```python
from build123d import *

# Parameters (mm, degrees)
F0_W     = 1400
F0_H     = 700
F0_W_2   = 420.8995199203
F0_H_2   = 620
F0_W_3   = 420
F0_H_3   = 350
F0_W_4   = 400
F0_H_4   = 600
F0_H_5   = 50
F1_DEPTH = 25
F2_DEPTH = 500
F3_START = 490
F3_DEPTH = 10


with BuildPart() as f1:
    # F0 (on Front) → F1 (new body)
    with BuildSketch(Plane.XZ):
        with Locations((0, 350)):
            Rectangle(F0_W, F0_H)
        with Locations((-450.4497599602, 350)):
            Rectangle(F0_W_2, F0_H_2, mode=Mode.SUBTRACT)
        with Locations((0, 350)):
            Rectangle(F0_W_3, F0_H_2, mode=Mode.SUBTRACT)
        with Locations((450, 350)):
            Rectangle(F0_W_3, F0_H_2, mode=Mode.SUBTRACT)
        with Locations((0, 875)):
            Rectangle(F0_W, F0_H_3)
        with Locations((0, 1275)):
            Rectangle(F0_W, F0_H_3)
        with Locations((0, 1675)):
            Rectangle(F0_W, F0_H_3)
        with Locations((-450.4497599602, 350)):
            Rectangle(F0_W_2, F0_H_2)
        with Locations((-450, 350)):
            Rectangle(F0_W_4, F0_H_4, mode=Mode.SUBTRACT)
        with Locations((450, 350)):
            Rectangle(F0_W_3, F0_H_2)
        with Locations((450, 350)):
            Rectangle(F0_W_4, F0_H_4, mode=Mode.SUBTRACT)
        with Locations((0, 350)):
            Rectangle(F0_W_3, F0_H_2)
        with Locations((0, 350)):
            Rectangle(F0_W_4, F0_H_4, mode=Mode.SUBTRACT)
        with Locations((450, 350)):
            Rectangle(F0_W_4, F0_H_4)
        with Locations((0, 350)):
            Rectangle(F0_W_4, F0_H_4)
        with Locations((-450, 350)):
            Rectangle(F0_W_4, F0_H_4)
        with Locations((0, 1075)):
            Rectangle(F0_W, F0_H_5)
        with Locations((0, 1475)):
            Rectangle(F0_W, F0_H_5)
        with Locations((0, 1875)):
            Rectangle(F0_W, F0_H_5)
    extrude(amount=F1_DEPTH)

    # F0 (on Front) → F2 (join)
    with BuildSketch(Plane.XZ):
        with Locations((0, 350)):
            Rectangle(F0_W, F0_H)
        with Locations((-450.4497599602, 350)):
            Rectangle(F0_W_2, F0_H_2, mode=Mode.SUBTRACT)
        with Locations((0, 350)):
            Rectangle(F0_W_3, F0_H_2, mode=Mode.SUBTRACT)
        with Locations((450, 350)):
            Rectangle(F0_W_3, F0_H_2, mode=Mode.SUBTRACT)
        with Locations((-450.4497599602, 350)):
            Rectangle(F0_W_2, F0_H_2)
        with Locations((-450, 350)):
            Rectangle(F0_W_4, F0_H_4, mode=Mode.SUBTRACT)
        with Locations((450, 350)):
            Rectangle(F0_W_3, F0_H_2)
        with Locations((450, 350)):
            Rectangle(F0_W_4, F0_H_4, mode=Mode.SUBTRACT)
        with Locations((0, 350)):
            Rectangle(F0_W_3, F0_H_2)
        with Locations((0, 350)):
            Rectangle(F0_W_4, F0_H_4, mode=Mode.SUBTRACT)
        with Locations((-450, 350)):
            Rectangle(F0_W_4, F0_H_4)
        with Locations((0, 350)):
            Rectangle(F0_W_4, F0_H_4)
        with Locations((450, 350)):
            Rectangle(F0_W_4, F0_H_4)
        with Locations((0, 1875)):
            Rectangle(F0_W, F0_H_5)
        with Locations((0, 1475)):
            Rectangle(F0_W, F0_H_5)
        with Locations((0, 1075)):
            Rectangle(F0_W, F0_H_5)
    extrude(amount=F2_DEPTH)

    # F0 (on Front) → F3 (cut)
    with BuildSketch(Plane.XZ.offset(F3_START)):
        with Locations((450, 350)):
            Rectangle(F0_W_3, F0_H_2)
        with Locations((450, 350)):
            Rectangle(F0_W_4, F0_H_4, mode=Mode.SUBTRACT)
        with Locations((0, 350)):
            Rectangle(F0_W_3, F0_H_2)
        with Locations((0, 350)):
            Rectangle(F0_W_4, F0_H_4, mode=Mode.SUBTRACT)
        with Locations((-450.4497599602, 350)):
            Rectangle(F0_W_2, F0_H_2)
        with Locations((-450, 350)):
            Rectangle(F0_W_4, F0_H_4, mode=Mode.SUBTRACT)
    extrude(amount=F3_DEPTH, mode=Mode.SUBTRACT)


solid = f1.part
```
The listing builds one solid part. Answer for the finished solid, in the listing's coordinates (mm). A direction names the side the tool comes from. Round coordinates to 2 decimals unless told otherwise and drop trailing zeros. Loops run counter-clockwise (first coordinate to the right, second up) from the corner with the lowest first, then second, coordinate; pieces in that order, holes last.
Q1. Which of the six approach directions +Z, -Z, +X, -X, +Y, -Y give full straight-line access (tool end or side, diameter ignored) to faces 1 (the face through (-10, -259, 1850)), 2 (the face through (-10, -246, 1900))?
Q2. Section B-B, the plane x = 172.5 is taken. Determine the outline of the cut face in (y, z).
Q3. For a pull along Z with two mould halves and no side action, classify faces 3 (the face through (-10, -246, 0)), 4 (the face through (447, -500, 354)), 5 (the face through (-10, -25, 877)) as released by +Z, released by -Z, zero draft, split by the parting line, or undercut.
Q4. Find the intervals of material crossed by line 1 (Z direction, x = 148, y = -193); line 2 (Y direction, x = -211.5, z = 1444), in increasing order.
Q5. Section C-C, the plane z = 756 is taken. Determine the outline of the cut face in (x, y).
Q6. Section A-A, the plane y = -326 is taken. Determine the outline of the cut face in (x, z), then the cut area to 3 significant figures.
Completed:
1. face 1: +X, -X, -Y
1. face 2: +Z, +X, -X, +Y, -Y
2. outline: (-500, 0) - (0, 0) - (0, 1900) - (-500, 1900) - (-500, 1850) - (-25, 1850) - (-25, 1500) - (-500, 1500) - (-500, 1450) - (-25, 1450) - (-25, 1100) - (-500, 1100) - (-500, 1050) - (-25, 1050) - (-25, 700) - (-500, 700) - (-500, 660) - (-490, 660) - (-490, 650) - (-500, 650) - (-500, 50) - (-490, 50) - (-490, 40) - (-500, 40) - close
3. face 3: released by -Z
3. face 4: zero draft
3. face 5: undercut
4. line 1: z = 0 to 700, 1050 to 1100, 1450 to 1500, 1850 to 1900
4. line 2: y = -25 to 0
5. outline: (-700, -25) - (700, -25) - (700, 0) - (-700, 0) - close
6. outline: (-700, 0) - (700, 0) - (700, 700) - (-700, 700) - close; (-700, 1050) - (700, 1050) - (700, 1100) - (-700, 1100) - close; (-700, 1450) - (700, 1450) - (700, 1500) - (-700, 1500) - close; (-700, 1850) - (700, 1850) - (700, 1900) - (-700, 1900) - close
6. area: 1,190,000 mm2
